Solid Edge part; units mm, degrees
sketch "Sketch1" plane through (0, 0, 0) normal (0, -1, 0) x (1, 0, 0)
  line L0 (-6.5, 3.5) -> (-6.5, -3.5)
  line L1 (-6.5, -3.5) -> (0, -3.5)
  line L2 (0, 3.5) -> (0, -3.5)
  line L3 (0, 3.5) -> (-6.5, 3.5)
revolve "RevolvedProtrusion1" add sketch "Sketch1" angle 360 about axis through (0, 0, 3.5) along (0, 0, -1)
sketch "Sketch2" plane through (0, 0, 3.5) normal (0, 0, 1) x (1, 0, 0)
  circle A0 centre (0, 0) radius 7.2656
extrude "Protrusion1" add sketch "Sketch2" along normal blind 1
sketch "Sketch3" plane through (0, 0, 0) normal (1, 0, 0) x (0, 1, 0)
  line L0 (0, 7.3) -> (0, -1.34)
  arc A0 (0, -1.34) -> (0, 7.3) centre (0, 2.98) cw
revolve "RevolvedProtrusion2" add sketch "Sketch3" angle 360 about axis through (0, 0, 7.3) along (0, 0, -1)
properties material "Alluminio 11/S EN AW 2011"
Can you work these out from the model? Positions are in its coordinate system, mm. A direction names the side the tool comes from. Round coordinates to 2 decimals unless told otherwise and drop trailing zeros. Loops run counter-clockwise (first coordinate to the right, second up) from the corner with the lowest first, then second, coordinate; pieces in that order, holes last. Notation, with made-up numbers: (65.25, 45.5) -> (96.25, 45.5) arc R28 cw to (96.25, 75.5) -> close; hole circle Ø3 at (20.25, 16.5). An arc over 180 degrees is marked (long way). One line per item, written item: value. Start each with the question number.
1. If we section it at D-D, the plane z = 4.75: Write out the boundary of the cut face in (x, y), then the cut area to 3 significant figures.
2. For pin 1 (5 mm diameter, centred on y = 3.5, z = 5, fed in from +X); pin 2 (1 mm diameter, centred on x = -5, z = 1, fed in from +Y); pin 3 (1 mm diameter, centred on x = 4.5, y = -5.5, fed in from +Z), each with a flat end and sliding along its axis, tell me the tip position at first contact or that it passes through.
3. If we section it at C-C, the plane z = 3: Write out the boundary of the cut face in (x, y), then the cut area to 3 significant figures.
4. If I drill on probe 1 along Z at (x, y) = (5.75, -0.75); probe 2 along X at (y, z) = (-0.25, -1.75); probe 3 along Z at (x, y) = (6, -3.5), over which ranges is the centre line in solid material (lowest first)?
5. If we section it at A-A, the plane y = 0: Write out the boundary of the cut face in (x, z), then the cut area to 3 significant figures.
6. For faces 1 (the cylindrical face through (5.158, -3.955, -0.049)), 2 (the flat face through (3, -3, 4.5)), 3 (the cylindrical face through (6.712, 2.783, 3.993)), which set-ups out of +Z, -Z, +X, -X, +Y, -Y let a thin tool reach every point of the face, with its end or its side?
Calculated:
1. outline: circle Ø7.88 at (0, 0)
1. area: 48.8 mm²
2. pin 1: stops at x = 7.19
2. pin 2: stops at y = 4.69
2. pin 3: stops at z = 4.5
3. outline: circle Ø13 at (0, 0)
3. area: 133 mm²
4. probe 1: z = -3.5 to 4.5
4. probe 2: x = -6.5 to 6.5
4. probe 3: z = 3.5 to 4.5
5. outline: (-7.27, 3.5) -> (-6.5, 3.5) -> (-6.5, -3.5) -> (6.5, -3.5) -> (6.5, 3.5) -> (7.27, 3.5) -> (7.27, 4.5) -> (4.04, 4.5) arc R4.32 ccw to (-4.04, 4.5) -> (-7.27, 4.5) -> close
5. area: 122 mm²
6. face 1: -Z
6. face 2: +Z
6. face 3: +Z, -Z
